```python
from build123d import *

# Parameters (mm, degrees)
SKETCH1_W           = 120
SKETCH1_H           = 34
BOSS_EXTRUDE1_DEPTH = 5
BOSS_EXTRUDE2_DEPTH = 2.5
SKETCH3_R           = 3.5
BOSS_EXTRUDE3_DEPTH = 16.75
SKETCH4_R           = 3.5
SKETCH4_R_2         = 3.175
CUT_EXTRUDE1_DEPTH  = 9.25
FILLET1_R           = 0.2


with BuildPart() as part:
    # Sketch1 → Boss-Extrude1 (new body)
    with BuildSketch(Plane(origin=(0, 0, 0), x_dir=(0, 0, -1), z_dir=(1, 0, 0))):
        with Locations((-60, 17)):
            Rectangle(SKETCH1_W, SKETCH1_H)
    extrude(amount=BOSS_EXTRUDE1_DEPTH)

    # Sketch2 → Boss-Extrude2 (add)
    with BuildSketch(Plane(origin=(5, 0, 0), x_dir=(0, 0, -1), z_dir=(1, 0, 0))):
        with BuildLine():
            ThreePointArc((-55, 17), (-56.464466094, 20.535533906), (-60, 22))
            Line((-60, 22), (-60, 12))
            ThreePointArc((-60, 12), (-56.464466094, 13.464466094), (-55, 17))
        make_face()
        with BuildLine():
            Line((-60, 12), (-60, 22))
            ThreePointArc((-60, 22), (-65, 17), (-60, 12))
        make_face()
    extrude(amount=BOSS_EXTRUDE2_DEPTH)

    # Sketch3 → Boss-Extrude3 (add)
    with BuildSketch(Plane(origin=(7.5, 0, 0), x_dir=(0, 0, -1), z_dir=(1, 0, 0))):
        with Locations((-60, 17)):
            Circle(SKETCH3_R)
    extrude(amount=BOSS_EXTRUDE3_DEPTH)

    # Sketch4 → Cut-Extrude1 (cut)
    with BuildSketch(Plane(origin=(24.25, 0, 0), x_dir=(0, 0, -1), z_dir=(1, 0, 0))):
        with Locations((-60, 17)):
            Circle(SKETCH4_R)
        with Locations((-60, 17)):
            Circle(SKETCH4_R_2, mode=Mode.SUBTRACT)
    extrude(amount=-CUT_EXTRUDE1_DEPTH, mode=Mode.SUBTRACT)

    # Fillet1
    fillet1_edges = [part.edges().sort_by_distance(p)[0] for p in [
        (5, 12, 60),
        (7.5, 17, 63.5),
    ]]
    fillet(fillet1_edges, radius=FILLET1_R)


solid = part.part
```
The listing builds one solid part. Answer for the finished solid, in the listing's coordinates (mm). A direction names the side the tool comes from. Coordinates: 2 decimals unless noted, no trailing zeros. Loops run counter-clockwise (first coordinate to the right, second up) from the corner with the lowest first, then second, coordinate; pieces in that order, holes last. Notation, with made-up numbers: (0, -29) - (43, -29) arc R22 cw to (43, -19) - close; hole circle Ø8 at (19, -37). An arc over 180 degrees is marked (long way). Write item = value, one per line.
1) Find the intervals of material crossed by line 1 along X through (y, z) = (4, 31.5); line 2 along Y through (x, z) = (18.25, 61), in increasing order.
Responses:
line_1 = 0 to 5
line_2 = 13.99 to 20.01
2) Section A-A (y = 30) is taken. Determine the outline of the cut face in (x, z).
Responses:
outline = (0, 0) - (5, 0) - (5, 120) - (0, 120) - close
3) This flat-tipped pin is pushed along its axis until it touches: P1, Ø6, axis at y = 8, z = 51.5, coming from the +X side. Where does it stop, or does it pass through?
Responses:
P1 = 5
4) Which of the six approach directions +Z, -Z, +X, -X, +Y, -Y give full straight-line access (tool end or side, diameter ignored) to faces 1 (the face through (24.25, 17, 60)), 2 (the face through (19.69, 17.95, 56.97))?
Responses:
face_1 = +Z, -Z, +X, +Y, -Y
face_2 = +X
